Job drawing, mm, ordinate dimensions from the low corner. One solid piece. A direction names the side the tool comes from. Round coordinates to 2 decimals unless told otherwise and drop trailing zeros. Loops run counter-clockwise (first coordinate to the right, second up) from the corner with the lowest first, then second, coordinate; pieces in that order, holes last.
1) Mould opens along X. For the marked faces 5, 6 and 7 say: +X half, -X half, draft (parallel to the pull), parting line (faces both ways), or undercut.
2) Drop flat-ended pins along their axis: P1, Ø11, axis at y = 29, z = 52, coming from the -X side (1 decimal); P2, Ø2, axis at x = 18.5, y = 64, coming from the -Z side; P3, Ø10, axis at y = 104.5, z = 82.5, coming from the +X side; P4, Ø13, axis at y = 114, z = 62.5, coming from the +X side. Give the stop position or say it passes through.
3) Probe line 1 (Y direction, x = 26, z = 5.5); line 2 (X direction, y = 26.5, z = 50.5) (1 decimal); line 3 (Z direction, x = 6.5, y = 56) (1 decimal). List the from-to ranges inside material, lowest first.
4) Band-saw the part on D-D, the plane x = 39.5. Write the cut outline in (y, z).
5) Band-saw the part on A-A, the plane z = 40.5. Write the cut outline in (x, y).
6) Band-saw the part on B-B, the plane x = 12. Write the cut outline in (y, z).
7) 3-axis set-ups, long thin cutter, end or side, ignore diameter. For the marked faces 1, 2, 3 and 4: which of +Z, -Z, +X, -X, +Y, -Y reach the whole face in a straight line?
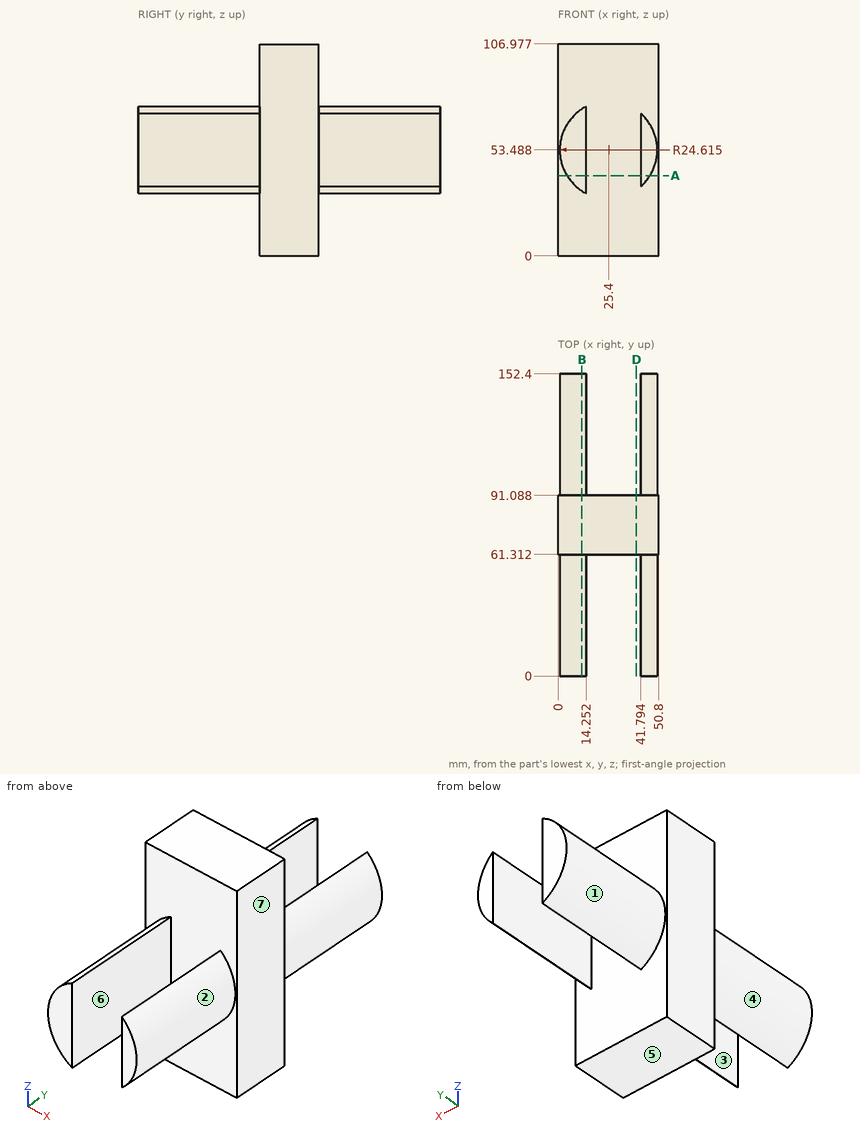
Reported:
1. face 5: draft
1. face 6: undercut
1. face 7: +X half
2. P1: stops at x = 0.8
2. P2: stops at z = 0
2. P3: passes through
2. P4: stops at x = 49.89
3. line 1: y = 61.31 to 91.09
3. line 2: x = 1 to 14.3, 41.8 to 49.8
3. line 3: z = 37.7 to 69.3
4. outline: (61.31, 0) - (91.09, 0) - (91.09, 106.98) - (61.31, 106.98) - close
5. outline: (0, 61.31) - (4.49, 61.31) - (4.49, 0) - (14.25, 0) - (14.25, 61.31) - (41.79, 61.31) - (41.79, 0) - (46.31, 0) - (46.31, 61.31) - (50.8, 61.31) - (50.8, 91.09) - (46.31, 91.09) - (46.31, 152.4) - (41.79, 152.4) - (41.79, 91.09) - (14.25, 91.09) - (14.25, 152.4) - (4.49, 152.4) - (4.49, 91.09) - (0, 91.09) - close
6. outline: (0, 32.84) - (61.31, 32.84) - (61.31, 0) - (91.09, 0) - (91.09, 32.84) - (152.4, 32.84) - (152.4, 74.14) - (91.09, 74.14) - (91.09, 106.98) - (61.31, 106.98) - (61.31, 74.14) - (0, 74.14) - close
7. face 1: -X, +Y
7. face 2: +X, -Y
7. face 3: +Z, -Z, -Y
7. face 4: -X, -Y
